Work out the finished part from the listing and answer in its coordinate system (mm). A direction names the side the tool comes from. Coordinates: 2 decimals unless noted, no trailing zeros. Write each loop counter-clockwise with the first axis right and the second up, starting at its lowest first coordinate (ties: lowest second). Pieces come first, ordered by that corner, then holes. Notation, with made-up numbers: (88, 21) - (110, 21) arc R23 ccw to (110, 30) - close; hole circle Ø1 at (14.5, -27.75). An arc over 180 degrees is marked (long way). Use a Markdown table: item, result. Add a question column.
(1) The part is cut by section D-D, the plane x = -35.5. Give the vertices of the cut face in (y, z) (3 decimals), then the cut area to 3 significant figures.
(2) For a pull along Y with two mould halves and no side action, classify faces 1 (the face through (35.366, 10.889, -44.406)), 2 (the face through (-1, -13, -44.45)), 3 (the face through (46.156, -12, -24)) as released by +Y, released by -Y, zero draft, split by the parting line, or undercut.
(3) A tool of negligible diameter and unlimited length cuts with its end or side. For faces 4 (the face through (33.456, 2, -44)), 5 (the face through (-35.366, 10.889, -44.406)), 6 (the face through (41, 5, -41.275)), 7 (the face through (39.895, -21.501, -45.214)), from which of +Z, -Z, +X, -X, +Y, -Y can it reach the whole face along a straight path? Write none if from no direction.
(4) The part is cut by section B-B, the plane z = -31.5. Give the vertices of the cut face in (x, y).
(5) Find the intervals of material crossed by line 1 (X direction, y = 6, z = -43); line 2 (X direction, y = -8.5, z = -18.5); line 3 (X direction, y = -6.5, z = -24.5), in increasing order. Write a range as from..to.
(6) The part is cut by section C-C, the plane x = 35. Give the vertices of the cut face in (y, z) (3 decimals).
(7) Given pin 1 Ø5 at (x, y) = (39.81, -31.75) entering from +Z (3 decimals); pin 2 Ø2 at (x, z) = (36.5, -37.5) entering from -Y; pin 3 Ø10 at (x, y) = (-29, -6.5) entering from -Z, each flat-ended and moving along its own axis, determine where each tip first touches the part or whether it passes through.
(8) The part is cut by section A-A, the plane y = 1.5. Give the vertices of the cut face in (x, z) (3 decimals), then the cut area to 3 significant figures.
from build123d import *

# Parameters (mm, degrees)
F1_DEPTH      = 25.4
F2_W          = 12.7
F2_H          = 6.35
F3_DEPTH      = 12.7
F3_DEPTH_BACK = 38.1
F4_R          = 6.34999
F5_W          = 19.05
F5_H          = 3.175
F6_DEPTH      = 92.3136190901
F7_W          = 66.9126190901
F7_H          = 3.175
F8_DEPTH      = 38.101
F9_R          = 2.54
F10_R         = 1.5875
F11_DEPTH     = 6.351


# Not quite as in the source:
# - a fillet or chamfer is up to 0.001 mm smaller than in the source, because OpenCascade refuses the exact size


with BuildPart() as f1:
    # F0 (on Front) → F1 (new body)
    with BuildSketch(Plane.XZ):
        with BuildLine():
            ThreePointArc((41.275, 0), (0, -41.275), (-41.275, 0))
            Line((-41.275, 0), (-46.156309545, 0))
            Line((-46.156309545, 0), (-46.156309545, -47.625))
            Line((-46.156309545, -47.625), (46.156309545, -47.625))
            Line((46.156309545, -47.625), (46.156309545, 0))
            Line((46.156309545, 0), (41.275, 0))
        make_face()
    extrude(amount=F1_DEPTH)

    # F2 (on face) → F3 (join, two sides)
    with BuildSketch(Plane.XZ.offset(25.4)) as f3_sk:
        with Locations((-39.806309545, -44.45)):
            Rectangle(F2_W, F2_H)
        with Locations((39.806309545, -44.45)):
            Rectangle(F2_W, F2_H)
    extrude(amount=F3_DEPTH)
    extrude(f3_sk.sketch, amount=-F3_DEPTH_BACK)

    # F4 (radius 6.35 in the source; OpenCascade refuses exactly that, so slightly less here)
    f4_edges = [f1.edges().sort_by_distance(p)[0] for p in [
        (-46.15631, 12.7, -44.45),
        (-33.45631, 12.7, -44.45),
        (-46.15631, -38.1, -44.45),
        (-33.45631, -38.1, -44.45),
        (33.45631, -38.1, -44.45),
        (46.15631, -38.1, -44.45),
        (33.45631, 12.7, -44.45),
        (46.15631, 12.7, -44.45),
    ]]
    fillet(f4_edges, radius=F4_R)

    # F5 (on face) → F6 (cut, through all)
    with BuildSketch(Plane(origin=(-46.156309545, 0, 0), x_dir=(0, -1, 0), z_dir=(-1, 0, 0))):
        with Locations((12.7, -46.0375)):
            Rectangle(F5_W, F5_H)
    extrude(amount=-F6_DEPTH, mode=Mode.SUBTRACT)

    # F7 (on face) → F8 (cut, through all)
    with BuildSketch(Plane.XZ.offset(25.4)):
        with Locations((0, -46.0375)):
            Rectangle(F7_W, F7_H)
    extrude(amount=-F8_DEPTH, mode=Mode.SUBTRACT)

    # F9
    f9_edges = [f1.edges().sort_by_distance(p)[0] for p in [
        (-39.80631, -22.225, -44.45),
        (-39.80631, -3.175, -44.45),
        (39.80631, -3.175, -44.45),
        (39.80631, -22.225, -44.45),
    ]]
    fillet(f9_edges, radius=F9_R)

    # F10 (on face) → F11 (cut, through all)
    with BuildSketch(Plane.XY.offset(-41.275)):
        with Locations((-39.806309545, -31.75)):
            Circle(F10_R)
        with Locations((-39.806309545, 6.35)):
            Circle(F10_R)
        with Locations((39.806309545, -31.75)):
            Circle(F10_R)
        with Locations((39.806309545, 6.35)):
            Circle(F10_R)
    extrude(amount=-F11_DEPTH, mode=Mode.SUBTRACT)


solid = f1.part
Model answer:
| question | item | result |
|---|---|---|
| 1 | outline | (-36.417, -47.625) - (-22.225, -47.625) - (-22.225, -46.99) arc R2.54 cw to (-19.685, -44.45) - (-5.715, -44.45) arc R2.54 cw to (-3.175, -46.99) - (-3.175, -47.625) - (11.017, -47.625) - (11.017, -41.275) - (0, -41.275) - (0, -21.056) - (-25.4, -21.056) - (-25.4, -41.275) - (-36.417, -41.275) - close |
| 1 | area | 757 mm^2 |
| 2 | face 1 | released by +Y |
| 2 | face 2 | undercut |
| 2 | face 3 | zero draft |
| 3 | face 4 | -Z, +Y |
| 3 | face 5 | +Z, -Z, +Y |
| 3 | face 6 | +Z, +X, -X, +Y |
| 3 | face 7 | -Z, +X, -X |
| 4 | outline | (-46.16, -25.4) - (-26.67, -25.4) - (-26.67, 0) - (-46.16, 0) - close; (26.67, -25.4) - (46.16, -25.4) - (46.16, 0) - (26.67, 0) - close |
| 5 | line 1 | -46.16..-41.35, -38.26..-33.46, 33.46..38.26, 41.35..46.16 |
| 5 | line 2 | -46.16..-36.9, 36.9..46.16 |
| 5 | line 3 | -46.16..-33.22, 33.22..46.16 |
| 6 | outline | (-35.9, -47.625) - (-22.225, -47.625) - (-22.225, -46.99) arc R2.54 cw to (-19.685, -44.45) - (-5.715, -44.45) arc R2.54 cw to (-3.175, -46.99) - (-3.175, -47.625) - (10.5, -47.625) - (10.5, -41.275) - (0, -41.275) - (0, -21.878) - (-25.4, -21.878) - (-25.4, -41.275) - (-35.9, -41.275) - close |
| 7 | pin 1 | z = -41.275 |
| 7 | pin 2 | y = -25.4 |
| 7 | pin 3 | z = -44.93 |
| 8 | outline | (-46.156, -47.625) - (-33.456, -47.625) - (-33.456, -41.275) - (-46.156, -41.275) - close; (33.456, -47.625) - (46.156, -47.625) - (46.156, -41.275) - (33.456, -41.275) - close |
| 8 | area | 161 mm^2 |
